Could you check a few things on this drawing? It's one solid part, dimensions in mm from its lowest x, y, z. A direction names the side the tool comes from. Give positions to 0.01 mm unless a question says otherwise; leave off trailing zeros. Order: outer loops, then holes, each group sorted by start corner. A loop starts at its lowest first (then second) coordinate and runs counter-clockwise, first axis right, second up. Notation, with made-up numbers: (39, 40) - (64, 40) arc R8 ccw to (64, 45) - close; hole circle Ø3 at (-37.75, -8.75). An arc over 180 degrees is marked (long way). Answer as CSV lines item,"result".
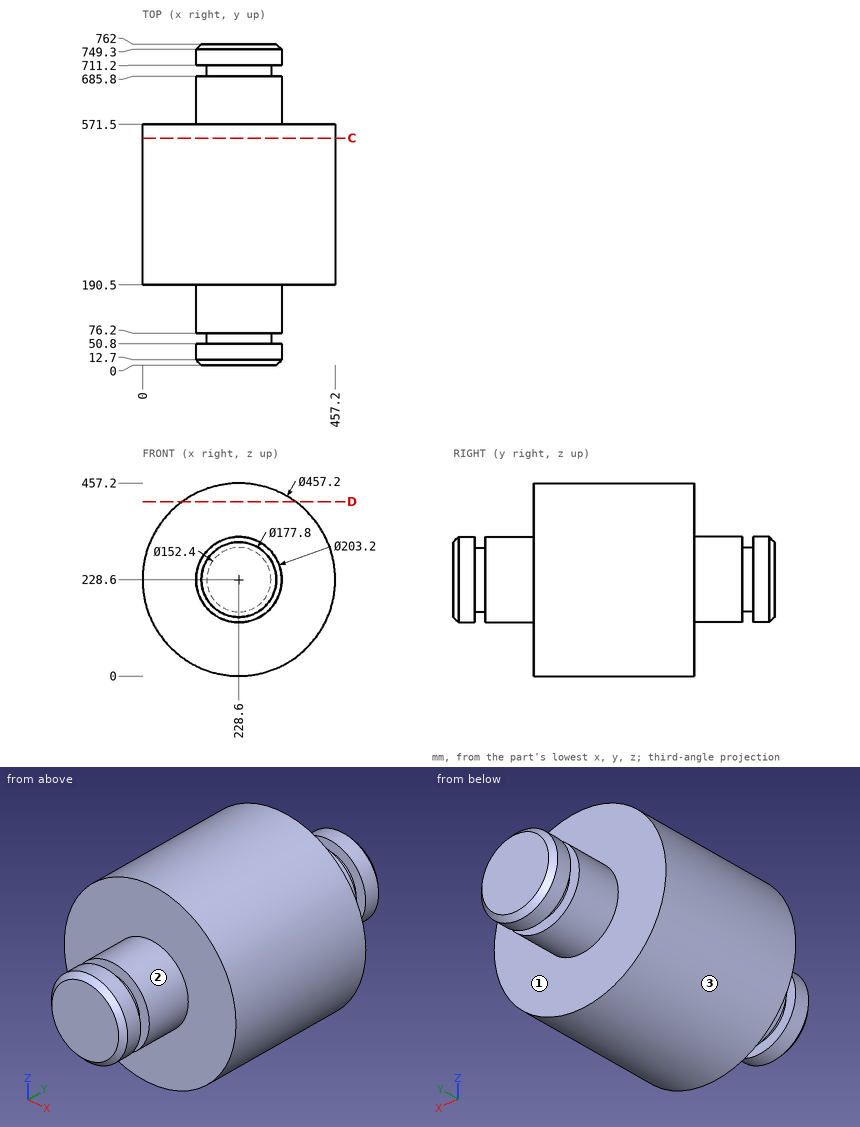
1) I want a section at C-C on y = 538.5. Write out the boundary of the cut face in (x, z), plus the area to 3 significant figures.
Answer block:
outline,"circle Ø457.2 at (228.6, 228.6)"
area,"164,000 mm2"
2) I want a section at D-D on z = 413.5. Write out the boundary of the cut face in (x, y), plus the area to 3 significant figures.
Answer block:
outline,"(94.18, 190.5) - (363.02, 190.5) - (363.02, 571.5) - (94.18, 571.5) - close"
area,"102,000 mm2"
3) I need wall thicknesses on line 1 along Y through (x, z) = (189, 150.5); line 2 along Y through (x, z) = (409, 273); line 3 along X through (y, z) = (434.5, 234.5). Which ranges of each line are inside material? Lowest first, please. Write a range as [from, to].
Answer block:
line 1,"[0, 50.8], [76.2, 685.8], [711.2, 762]"
line 2,"[190.5, 571.5]"
line 3,"[0.08, 457.12]"
4) Which directions (+Z, -Z, +X, -X, +Y, -Y) give clear straight access to the entire face, cutting with the end or side of a thin tool? Please do the marked faces 1, 2 and 3.
Answer block:
face 1,"+Y"
face 2,"-Y"
face 3,"+Y, -Y"
5) I'm going to push flat-ended pins straight in: P1, Ø12, axis at x = 88, y = 476.5, coming from the +Z side; P2, Ø10, axis at x = 246.5, z = 394, coming from the +Y side; P3, Ø1.5, axis at x = 100, z = 177, coming from the -Y side. Where does each tip first touch, or does it pass through?
Answer block:
P1,"z = 413.37"
P2,"y = 571.5"
P3,"y = 190.5"
